from build123d import *

# Parameters (mm, degrees)
SKETCH1_R           = 2.54
BOSS_EXTRUDE1_DEPTH = 3.175


with BuildPart() as part:
    # Sketch1 → Boss-Extrude1 (new body)
    with BuildSketch(Plane.XY):
        with BuildLine():
            Line((267.156088922, 46.92365038), (279.140387862, 34.939351441))
            Line((279.140387862, 34.939351441), (281.571044282, 23.781894278))
            ThreePointArc((281.571044282, 23.781894278), (284.344053276, 19.790554308), (289.127170298, 18.929064213))
            Line((289.127170298, 18.929064213), (317.240211958, 25.053501369))
            ThreePointArc((317.240211958, 25.053501369), (321.231551928, 27.826510362), (322.093042023, 32.609627384))
            Line((322.093042023, 32.609627384), (317.287210275, 54.669866506))
            ThreePointArc((317.287210275, 54.669866506), (314.35957702, 61.811763931), (309.165828873, 67.521642695))
            Line((309.165828873, 67.521642695), (294.956987541, 78.507489408))
            ThreePointArc((294.956987541, 78.507489408), (284.701481461, 158.676495857), (364.87048791, 168.932001937))
            Line((364.87048791, 168.932001937), (379.079329242, 157.946155224))
            ThreePointArc((379.079329242, 157.946155224), (412.294400675, 165.089560033), (399.659420331, 196.627259288))
            Line((399.659420331, 196.627259288), (161.950324224, 275.333486261))
            ThreePointArc((161.950324224, 275.333486261), (134.2512057, 280.394583932), (106.226730954, 277.658767447))
            Line((106.226730954, 277.658767447), (-8.234725559, 250.092638572))
            ThreePointArc((-8.234725559, 250.092638572), (-34.925, 211.753723054), (0, 180.729739303))
            Line((0, 180.729739303), (91.265902063, 180.729739303))
            Line((91.265902063, 180.729739303), (155.941245852, 180.729739303))
            Line((155.941245852, 180.729739303), (163.107951031, 150.971788271))
            Line((163.107951031, 150.971788271), (267.156088922, 46.92365038))
        make_face()
        with Locations((392.673620981, 175.528699327)):
            Circle(SKETCH1_R, mode=Mode.SUBTRACT)
        with Locations((295.571537134, 49.939098592)):
            Circle(SKETCH1_R, mode=Mode.SUBTRACT)
        with Locations((0, 215.9)):
            Circle(SKETCH1_R, mode=Mode.SUBTRACT)
    extrude(amount=BOSS_EXTRUDE1_DEPTH)


solid = part.part
Source: CAD feature listing. Evaluate the final solid. Frame: model axes, mm. A direction names the side the tool comes from. Round coordinates to 2 decimals unless told otherwise and drop trailing zeros. Loops run counter-clockwise (first coordinate to the right, second up) from the corner with the lowest first, then second, coordinate; pieces in that order, holes last. Notation, with made-up numbers: M 66,-21.75 L 117,-21.75 A19 cw 117,15.25 Z; hole C -2,21 d3. An arc over 180 degrees is marked long. Return JSON: item names as keys, results as strings. Group by question number.
1. Pin query (flat end, axial travel): pin 1 (4.5 mm diameter, centred on x = 392.67, y = 175.53, fed in from +Z); pin 2 (1.5 mm diameter, centred on y = 90, z = 1, fed in from +X); pin 3 (1 mm diameter, centred on x = 88.5, z = 1.5, fed in from -Y). Return the tip coordinate at first contact, or that it passes through.
2. Section query C-C on y = 207. Output: boundary loops of the cut face in (x, z) (3 decimals), and give its area (3 significant figures).
3. Section query A-A on z = 1.2. State how many separate pieces and enclosed holes the cut face has, and give its area (3 significant figures).
4. Material intervals for line 1 along Y through (x, z) = (300, 2.05); line 2 along Y through (x, z) = (368, 2.5); line 3 along Y through (x, z) = (208.5, 1.1), sorted ascending. Write a range as from..to.
5. Reachability of faces 1 (the face through (302.16, 72.94, 1.57)), 2 (the face through (371.875, 163.516, 1.565)), 3 (the face through (189, 189, 0)) from +Z, -Z, +X, -X, +Y, -Y: full face, straight path, thin tool, end or side. Return the list, or none.
6. Mould query, pull axis Y, two halves, no side actions, for faces 4 (the face through (314.417, 61.72, 1.565)), 5 (the face through (-35, 212.46, 1.57)), 6 (the face through (49.8, 264.07, 1.57)). Classes: released by +Y, released by -Y, zero draft, split by the parting line, or undercut.
7. Section query B-B on x = 89. Output: boundary loops of the cut face in (y, z) (3 decimals), and give its area (3 significant figures).
Checks:
{
 "1": {"pin 1": "passes through", "pin 2": "stops at x = 284.33", "pin 3": "stops at y = 180.73"},
 "2": {"outline": "M -34.026,0 L 368.332,0 L 368.332,3.175 L -34.026,3.175 Z", "area": "1,280 mm²"},
 "3": {"separate pieces": "1", "enclosed holes": "3", "area": "43,500 mm²"},
 "4": {"line 1": "y = 21.3..74.61, 172.42..229.62", "line 2": "y = 166.51..207.11", "line 3": "y = 105.58..259.92"},
 "5": {"face 1": "+Z, -Z, +X", "face 2": "+Z, -Z, -Y", "face 3": "-Z, +X, -X, +Y, -Y"},
 "6": {"face 4": "undercut", "face 5": "split by the parting line", "face 6": "released by +Y"},
 "7": {"outline": "M 180.73,0 L 273.51,0 L 273.51,3.175 L 180.73,3.175 Z", "area": "295 mm²"}
}
